Read the model definition and answer for the solid it produces. Units are mm, in the model's axes. A direction names the side the tool comes from. Coordinates: 2 decimals unless noted, no trailing zeros. Loops run counter-clockwise (first coordinate to the right, second up) from the corner with the lowest first, then second, coordinate; pieces in that order, holes last. Notation, with made-up numbers: (2, 50) - (7, 50) arc R27 cw to (7, 78) - close; hole circle Ø5 at (71, 6). An arc over 180 degrees is marked (long way). Use one line per item in the form item = value. Start each with the question number.
1) A cutting plane is placed at C-C (x = -12). Give the vertices of the cut face in (y, z).
2) A cutting plane is placed at D-D (z = 0.5). Give the vertices of the cut face in (x, y).
3) The mould has two halves that part along X. Classify faces 1 (the face through (0, -18, 1.5)), 2 (the face through (13.9, -19.93, 1.83)), 3 (the face through (-12, -6, 7.5)): released by +X, released by -X, zero draft, split by the parting line, or undercut.
4) A cutting plane is placed at B-B (y = -10). Give the vertices of the cut face in (x, z).
5) Consider line 1 (Y direction, x = -12, z = 5.5); line 2 (Y direction, x = 0, z = -0.95); line 3 (Y direction, x = 0, z = -3.15). Determine where each line is inside the solid, lowest interval first.
6) Each of these flat-tipped pins is pushed along its axis until it touches: P1, Ø4, axis at x = 0, y = 10, coming from the +Z side; P2, Ø1, axis at x = -13, y = 9.5, coming from the +Z side; P3, Ø5.5, axis at x = 0, y = 0, coming from the +Z side. Where does it stop, or does it pass through?
7) A cutting plane is placed at A-A (z = 6). Give the vertices of the cut face in (x, y).
8) Which of the six approach directions +Z, -Z, +X, -X, +Y, -Y give full straight-line access (tool end or side, diameter ignored) to faces 4 (the face through (12.53, -19.02, 3.7)), 5 (the face through (-6, -18, 5)), 6 (the face through (11, 0, 7.5)), 7 (the face through (-2.5, 18, 5))?
from build123d import *

# Parameters (mm, degrees)
F0_W           = 29
F0_H           = 41
F0_R           = 1.15
F0_W_2         = 19
F0_H_2         = 31
F1_DEPTH       = 7.5
F2_W           = 29
F2_H           = 41
F2_R           = 1.15
F2_W_2         = 19
F2_H_2         = 31
F3_DEPTH       = 4
F4_W           = 12
F4_H           = 5
F4_W_2         = 5
F5_DEPTH       = 6
F6_R           = 2
F8_D           = 2.9
F8_CBORE_D     = 5.5
F8_CBORE_DEPTH = 2.5
F9_W           = 5
F9_H           = 3.5
F10_DEPTH      = 5


with BuildPart() as f1:
    # F0 (on Top) → F1 (new body)
    with BuildSketch(Plane.XY):
        Rectangle(F0_W, F0_H)
        with Locations((-12, -18)):
            Circle(F0_R, mode=Mode.SUBTRACT)
        with Locations((12, -18)):
            Circle(F0_R, mode=Mode.SUBTRACT)
        with Locations((-12, 18)):
            Circle(F0_R, mode=Mode.SUBTRACT)
        Rectangle(F0_W_2, F0_H_2, mode=Mode.SUBTRACT)
        with Locations((12, 18)):
            Circle(F0_R, mode=Mode.SUBTRACT)
    extrude(amount=F1_DEPTH)

    # F2 (on face) → F3 (join)
    with BuildSketch(Plane(origin=(0, 0, 0), x_dir=(1, 0, 0), z_dir=(0, 0, -1))):
        Rectangle(F2_W, F2_H)
        with Locations((-12, -18)):
            Circle(F2_R, mode=Mode.SUBTRACT)
        with Locations((12, -18)):
            Circle(F2_R, mode=Mode.SUBTRACT)
        with Locations((-12, 18)):
            Circle(F2_R, mode=Mode.SUBTRACT)
        Rectangle(F2_W_2, F2_H_2, mode=Mode.SUBTRACT)
        with Locations((12, 18)):
            Circle(F2_R, mode=Mode.SUBTRACT)
        with Locations((-12, 18)):
            Circle(F2_R)
        with Locations((12, 18)):
            Circle(F2_R)
        with Locations((-12, -18)):
            Circle(F2_R)
        Rectangle(F2_W_2, F2_H_2)
        with Locations((12, -18)):
            Circle(F2_R)
    extrude(amount=F3_DEPTH)

    # F4 (on face) → F5 (cut)
    with BuildSketch(Plane.XY.offset(7.5)):
        with Locations((0, -18)):
            Rectangle(F4_W, F4_H)
        with Locations((0, 18)):
            Rectangle(F4_W_2, F4_H)
    extrude(amount=-F5_DEPTH, mode=Mode.SUBTRACT)

    # F6
    f6_edges = [f1.edges().sort_by_distance(p)[0] for p in [
        (-14.5, 20.5, 1.75),
        (14.5, 20.5, 1.75),
        (14.5, -20.5, 1.75),
        (-14.5, -20.5, 1.75),
    ]]
    fillet(f6_edges, radius=F6_R)

    # F8 (through all)
    with Locations(Plane.XY):
        with Locations((0, 10), (0, -10)):
            CounterBoreHole(F8_D / 2, F8_CBORE_D / 2, F8_CBORE_DEPTH)

    # F9 (on face) → F10 (cut)
    with BuildSketch(Plane.XY.offset(7.5)):
        with Locations((-12, 10.25)):
            Rectangle(F9_W, F9_H)
    extrude(amount=-F10_DEPTH, mode=Mode.SUBTRACT)


solid = f1.part
Found:
q1.outline = (-20.5, -4) - (20.5, -4) - (20.5, 7.5) - (19.15, 7.5) - (19.15, 0) - (16.85, 0) - (16.85, 7.5) - (12, 7.5) - (12, 2.5) - (8.5, 2.5) - (8.5, 7.5) - (-16.85, 7.5) - (-16.85, 0) - (-19.15, 0) - (-19.15, 7.5) - (-20.5, 7.5) - close
q2.outline = (-14.5, -18.5) arc R2 ccw to (-12.5, -20.5) - (12.5, -20.5) arc R2 ccw to (14.5, -18.5) - (14.5, 18.5) arc R2 ccw to (12.5, 20.5) - (-12.5, 20.5) arc R2 ccw to (-14.5, 18.5) - close; hole circle Ø2.3 at (-12, -18); hole circle Ø2.3 at (-12, 18); hole (-9.5, -15.5) - (9.5, -15.5) - (9.5, 15.5) - (-9.5, 15.5) - close; hole circle Ø2.3 at (12, -18); hole circle Ø2.3 at (12, 18)
q3.face_1 = undercut
q3.face_2 = released by +X
q3.face_3 = zero draft
q4.outline = (-14.5, -4) - (-1.45, -4) - (-1.45, -2.5) - (-2.75, -2.5) - (-2.75, 0) - (-9.5, 0) - (-9.5, 7.5) - (-14.5, 7.5) - close; (1.45, -4) - (14.5, -4) - (14.5, 7.5) - (9.5, 7.5) - (9.5, 0) - (2.75, 0) - (2.75, -2.5) - (1.45, -2.5) - close
q5.line_1 = -20.5 to -19.15, -16.85 to 8.5, 12 to 16.85, 19.15 to 20.5
q5.line_2 = -20.5 to -12.75, -7.25 to 7.25, 12.75 to 20.5
q5.line_3 = -20.5 to -11.45, -8.55 to 8.55, 11.45 to 20.5
q6.P1 = -2.5
q6.P2 = 2.5
q6.P3 = 0
q7.outline = (-14.5, -18.5) arc R2 ccw to (-12.5, -20.5) - (-6, -20.5) - (-6, -15.5) - (-9.5, -15.5) - (-9.5, 8.5) - (-14.5, 8.5) - close; (-14.5, 12) - (-9.5, 12) - (-9.5, 15.5) - (-2.5, 15.5) - (-2.5, 20.5) - (-12.5, 20.5) arc R2 ccw to (-14.5, 18.5) - close; (2.5, 15.5) - (9.5, 15.5) - (9.5, -15.5) - (6, -15.5) - (6, -20.5) - (12.5, -20.5) arc R2 ccw to (14.5, -18.5) - (14.5, 18.5) arc R2 ccw to (12.5, 20.5) - (2.5, 20.5) - close; hole circle Ø2.3 at (-12, -18); hole circle Ø2.3 at (-12, 18); hole circle Ø2.3 at (12, -18); hole circle Ø2.3 at (12, 18)
q8.face_4 = +Z
q8.face_5 = +Z, -Y
q8.face_6 = +Z, +X, -X, +Y, -Y
q8.face_7 = +Z, +Y, -Y
